Source: three-view drawing plus pictorial views. Frame: mm from the lowest corner of the part. A direction names the side the tool comes from. Give positions to 0.01 mm unless a question says otherwise; leave off trailing zeros. Write each loop counter-clockwise with the first axis right and the second up, starting at its lowest first coordinate (ties: lowest second). Pieces come first, ordered by that corner, then holes.
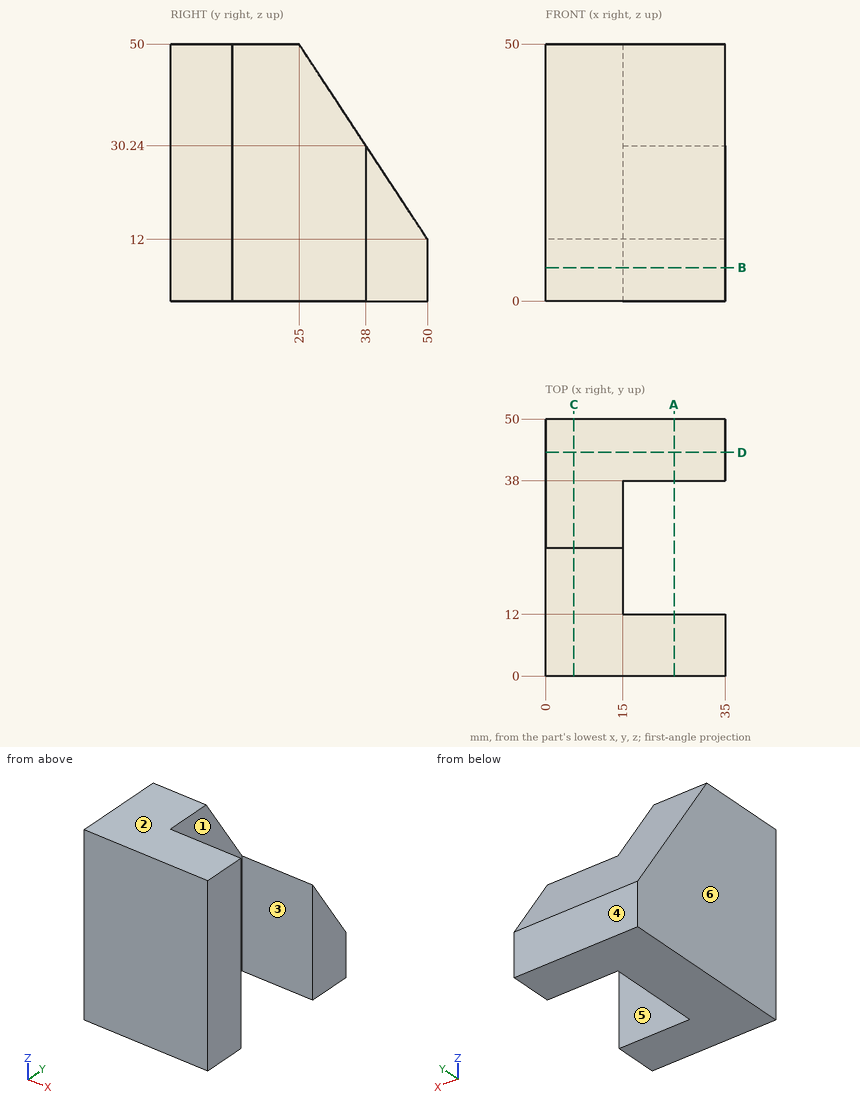
Q1. Section B-B on z = 6.5. Output: boundary loops of the cut face in (x, y), plus the area to 3 significant figures.
Filled sheet:
outline: (0, 0) - (35, 0) - (35, 12) - (15, 12) - (15, 38) - (35, 38) - (35, 50) - (0, 50) - close
area: 1,230 mm2
Q2. Section D-D on y = 43.5. Output: boundary loops of the cut face in (x, z).
Filled sheet:
outline: (0, 0) - (35, 0) - (35, 21.88) - (0, 21.88) - close
Q3. Section C-C on x = 5.5. Output: boundary loops of the cut face in (y, z).
Filled sheet:
outline: (0, 0) - (50, 0) - (50, 12) - (25, 50) - (0, 50) - close
Q4. Access query for the marked faces 5 and 6. Directions: +Z, -Z, +X, -X, +Y, -Y. A direction counts if a zero-diameter tool reaches every point of the face in a straight line with its end or side. Return the directions, or none.
Filled sheet:
face 5: +Z, -Z, +X
face 6: +Z, -Z, -X, +Y, -Y
Q5. Pin query (flat end, axial travel): P1, Ø16, axis at x = 23, z = 26.5, coming from the +Y side; P2, Ø3, axis at x = 22.5, z = 17, coming from the +Y side; P3, Ø5, axis at x = 21, z = 13.5, coming from the +Y side; P4, Ø5, axis at x = 19.5, y = 22, coming from the -Z side. Return the tip coordinate at first contact, or that it passes through.
Filled sheet:
P1: stops at y = 45.72
P2: stops at y = 47.7
P3: stops at y = 50
P4: passes through
Q6. Section A-A on x = 25. Output: boundary loops of the cut face in (y, z).
Filled sheet:
outline: (0, 0) - (12, 0) - (12, 50) - (0, 50) - close; (38, 0) - (50, 0) - (50, 12) - (38, 30.24) - close
Q7. Ray query, line 1 along Y through (x, z) = (17, 12); line 2 along X through (y, z) = (21.5, 17); line 3 along Y through (x, z) = (23.5, 45.5). Return the intervals inside material, ascending.
Filled sheet:
line 1: y = 0 to 12, 38 to 50
line 2: x = 0 to 15
line 3: y = 0 to 12
Q8. Pull-direction query (Y, two-part tool) for the marked faces 1, 2, 3 and 4; classes: released by +Y, released by -Y, zero draft, split by the parting line, or undercut.
Filled sheet:
face 1: undercut
face 2: zero draft
face 3: undercut
face 4: released by +Y
